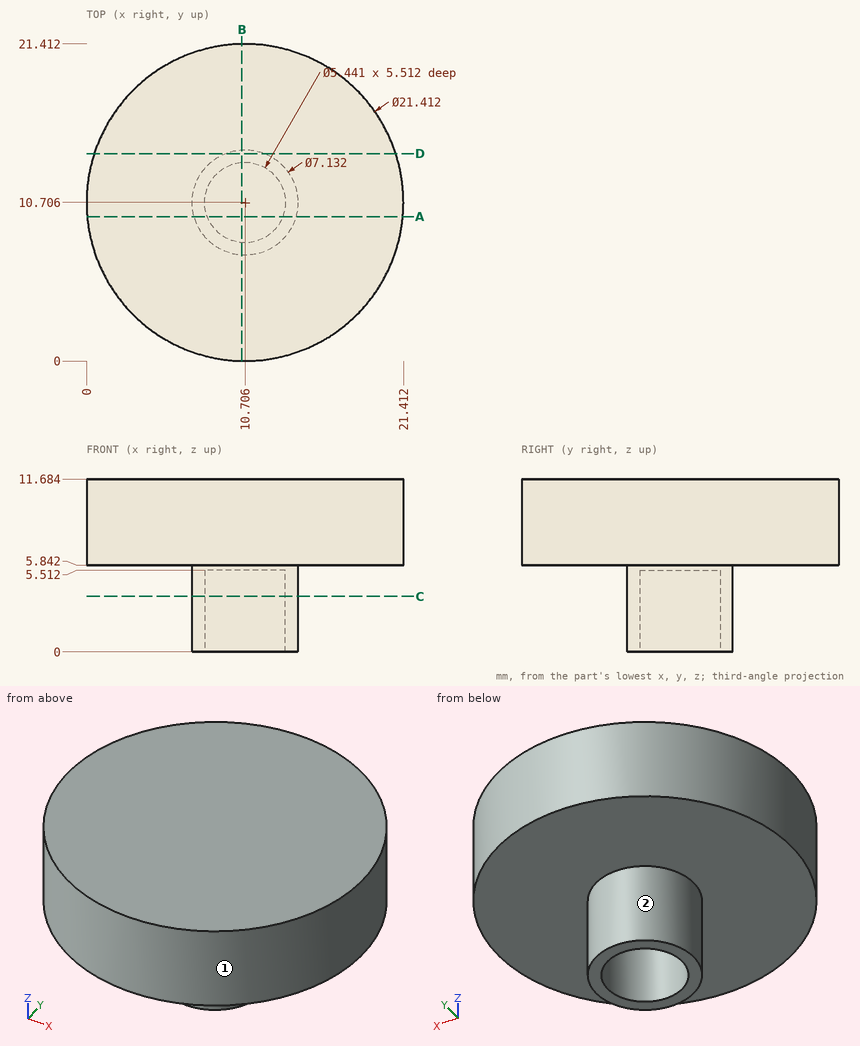
Drawing for the job (mm, zero at the part's lowest x, y, z). A direction names the side the tool comes from. Round coordinates to 2 decimals unless told otherwise and drop trailing zeros. Write each loop counter-clockwise with the first axis right and the second up, starting at its lowest first coordinate (ties: lowest second). Pieces come first, ordered by that corner, then holes. Notation, with made-up numbers: (81.5, -2.5) - (132.5, -2.5) arc R5 cw to (132.5, 3.5) - close; hole circle Ø7 at (19, 0). An arc over 180 degrees is marked (long way). Write item = value, one per line. Start each with the question number.
Q1. Probe L1, parallel to Z at x = 9.5, y = 19; L2, parallel to Y at x = 4.75, z = 8.75; L3, parallel to Y at x = 16.5, z = 11.25 (1 decimal). List the from-to ranges inside material, lowest first. Write a range as from..to.
Q2. Band-saw the part on A-A (y = 9.75). Give the cut face in (x, z).
Q3. Band-saw the part on B-B (x = 10.5). Give the cut face in (y, z) (1 decimal), then the cut area to 3 significant figures.
Q4. Band-saw the part on D-D (y = 14). Give the cut face in (x, z), then the cut area to 3 significant figures.
Q5. Band-saw the part on C-C (z = 3.75). Give the cut face in (x, y).
Q6. Drop flat-ended pins along their axis: pin 1 (2.5 mm diameter, centred on x = 10.5, y = 10.5, fed in from -Z); pin 2 (1 mm diameter, centred on x = 3.5, y = 15.5, fed in from -Z); pin 3 (1 mm diameter, centred on y = 16.5, z = 7.5, fed in from -X). Give the stop position or say it passes through.
Q7. Which spindle directions (+Z, -Z, +X, -X, +Y, -Y) get a long thin tool onto all of the face, cutting with end or side? Do the marked faces 1 and 2. Say none if no direction does.
Answers below:
q1.L1 = 5.84..11.68
q1.L2 = 1.81..19.6
q1.L3 = 1.7..19.7
q2.outline = (0.04, 5.84) - (7.27, 5.84) - (7.27, 0) - (8.16, 0) - (8.16, 5.51) - (13.25, 5.51) - (13.25, 0) - (14.14, 0) - (14.14, 5.84) - (21.37, 5.84) - (21.37, 11.68) - (0.04, 11.68) - close
q3.outline = (0, 5.8) - (7.1, 5.8) - (7.1, 0) - (8, 0) - (8, 5.5) - (13.4, 5.5) - (13.4, 0) - (14.3, 0) - (14.3, 5.8) - (21.4, 5.8) - (21.4, 11.7) - (0, 11.7) - close
q3.area = 137 mm2
q4.outline = (0.52, 5.84) - (9.34, 5.84) - (9.34, 0) - (12.07, 0) - (12.07, 5.84) - (20.89, 5.84) - (20.89, 11.68) - (0.52, 11.68) - close
q4.area = 135 mm2
q5.outline = circle Ø7.13 at (10.71, 10.71); hole circle Ø5.44 at (10.71, 10.71)
q6.pin_1 = 5.51
q6.pin_2 = 5.84
q6.pin_3 = 1.4
q7.face_1 = +Z, -Z
q7.face_2 = -Z
